```python
from build123d import *

# Parameters (mm, degrees)
SKETCH_1_R       = 2.5
EXTRUDE_1_DEPTH  = 2
SKETCH_2_R       = 1.95
EXTRUDE_2_DEPTH  = 70
CHAMFER_1_SIZE   = 1.5
CHAMFER_1_SIZE_2 = 2.598076211


with BuildPart() as part:
    # 草图1 → 凸台-拉伸1 (new body)
    with BuildSketch(Plane(origin=(0, 0, 0), x_dir=(1, 0, 0), z_dir=(0, 1, 0))):
        with Locations(Location((0, 0, 0), (0, 0, 270))):
            Circle(SKETCH_1_R)
    extrude(amount=EXTRUDE_1_DEPTH)

    # 草图2 → 凸台-拉伸2 (add)
    with BuildSketch(Plane.XZ):
        with Locations(Location((0, 0, 0), (0, 0, 270))):
            Circle(SKETCH_2_R)
    extrude(amount=EXTRUDE_2_DEPTH)

    # 倒角1
    # the kernel refuses this chamfer: 2.598076211, 1.5 mm, written as the material it adds along each edge
    with BuildSketch(Plane(origin=(0, 0, 0), x_dir=(0, 0, -1), z_dir=(-1, 0, 0))) as chamfer_1_piece_1_section:
        Polygon((1.95 + CHAMFER_1_SIZE, 0), (1.95, CHAMFER_1_SIZE_2), (1.95, 0), align=None)
    chamfer_1_piece_1 = revolve(axis=Axis((0, 0, 0), (0, -1, 0)), mode=Mode.PRIVATE)
    chamfer_1_piece_1 = chamfer_1_piece_1 & Plane(origin=(0, -2.153550613, 0), x_dir=(0, 0, 1), z_dir=(0, -1, 0)) * Cylinder(2.5, 14, mode=Mode.PRIVATE)
    add(chamfer_1_piece_1)


solid = part.part
```
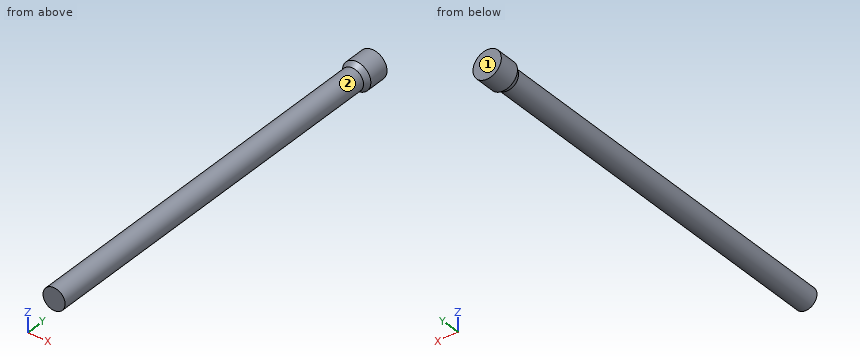
Build history of the part. All positions in model axes, mm. Face numbers are marked on the shaded views. A direction names the side the tool comes from. Give positions to 0.01 mm unless a question says otherwise; leave off trailing zeros. Loops run counter-clockwise (first coordinate to the right, second up) from the corner with the lowest first, then second, coordinate; pieces in that order, holes last.
Item 1: Slice it at A-A, the plane x = 0. List the corners of the cut face in (y, z).
Answers follow:
outline: (-70, -1.95) - (-2.6, -1.95) - (-1.65, -2.5) - (2, -2.5) - (2, 2.5) - (-1.65, 2.5) - (-2.6, 1.95) - (-70, 1.95) - close
Item 2: Drill centre lines: line 1 (Z direction, x = 0.05, y = -10.5); line 2 (X direction, y = -25.5, z = -0.2); line 3 (Y direction, x = -2.1, z = 0.55). Where is each one in solid material? Low to high.
Answers follow:
line 1: z = -1.95 to 1.95
line 2: x = -1.94 to 1.94
line 3: y = -2.22 to 2
Item 3: Flat gauge pins, fed straight in: pin 1 (2 mm diameter, centred on y = -45.5, z = -1, fed in from +X); pin 2 (3 mm diameter, centred on x = 1.5, y = -50.5, fed in from -Z); pin 3 (2 mm diameter, centred on y = -40, z = -1, fed in from -X). Where does each tip first touch, or does it go through?
Answers follow:
pin 1: stops at x = 1.95
pin 2: stops at z = -1.95
pin 3: stops at x = -1.95
Item 4: Slice it at B-B, the plane z = 0. List the corners of the cut face in (x, y).
Answers follow:
outline: (-2.5, -1.65) - (-1.95, -2.6) - (-1.95, -70) - (1.95, -70) - (1.95, -2.6) - (2.5, -1.65) - (2.5, 2) - (-2.5, 2) - close
Item 5: Which spindle directions (+Z, -Z, +X, -X, +Y, -Y) get a long thin tool onto all of the face, cutting with end or side? Do the marked faces 1 and 2. Say none if no direction does.
Answers follow:
face 1: +Z, -Z, +X, -X, +Y
face 2: -Y
Item 6: Slice it at C-C, the plane y = -18.5. List the corners of the cut face in (x, z).
Answers follow:
outline: circle Ø3.9 at (0, 0)
